Autodesk Inventor part; units mm, degrees
ref_plane "YZ Plane" through (0, 0, 0) normal (1, 0, 0) x (0, 1, 0)
ref_plane "XZ Plane" through (0, 0, 0) normal (0, 1, 0) x (-1, 0, 0)
ref_plane "XY Plane" through (0, 0, 0) normal (0, 0, 1) x (1, 0, 0)
sketch "Sketch1" plane through (0, 0, 0) normal (0, 1, 0) x (-1, 0, 0)
  line L0 (15.875, 38.1) -> (-15.875, 38.1)
  line L1 (-25.4, 28.575) -> (-25.4, -28.575)
  line L2 (-15.875, -38.1) -> (15.875, -38.1)
  line L3 (25.4, -28.575) -> (25.4, 28.575)
  line L4 (25.4, 38.1) -> (-25.4, -38.1) construction
  line L5 (-25.4, 38.1) -> (25.4, -38.1) construction
  arc A0 (15.875, -38.1) -> (25.4, -28.575) centre (15.875, -28.575) ccw
  arc A1 (25.4, 28.575) -> (15.875, 38.1) centre (15.875, 28.575) ccw
  arc A2 (-15.875, 38.1) -> (-25.4, 28.575) centre (-15.875, 28.575) ccw
  arc A3 (-25.4, -28.575) -> (-15.875, -38.1) centre (-15.875, -28.575) ccw
  line L6 (15.875, -34.925) -> (-15.875, -34.925)
  arc A4 (-22.225, -28.575) -> (-15.875, -34.925) centre (-15.875, -28.575) ccw
  line L7 (-22.225, -28.575) -> (-22.225, 28.575)
  arc A5 (-15.875, 34.925) -> (-22.225, 28.575) centre (-15.875, 28.575) ccw
  line L8 (-15.875, 34.925) -> (15.875, 34.925)
  arc A6 (22.225, 28.575) -> (15.875, 34.925) centre (15.875, 28.575) ccw
  line L9 (22.225, 28.575) -> (22.225, -28.575)
  arc A7 (15.875, -34.925) -> (22.225, -28.575) centre (15.875, -28.575) ccw
  point P0 (0, 0)
  dimension "d0" = 76.2
  dimension "d1" = 50.8
  dimension "d2" = 9.525
  dimension "d3" = 3.175
extrude "Extrusion1" add sketch "Sketch1" along normal blind 955.1356
sketch "Sketch2" plane through (-25.4, 0, -28.575) normal (-1, 0, 0) x (0, 0, 1)
  line L0 (0, 955.1356) -> (-9.525, 955.1356)
  line L1 (-9.525, 955.1356) -> (66.675, 471.8415)
  line L2 (66.675, 0) -> (66.675, 955.1356)
  line L3 (66.675, 471.8415) -> (66.675, 955.1356)
  line L4 (66.675, 955.1356) -> (-9.525, 955.1356)
  line L5 (-9.525, 0) -> (-9.525, 955.1356)
  point P0 (28.575, 0)
  dimension "d6" = 8.96
extrude "Extrusion2" cut sketch "Sketch2" against normal through all
equation "\"d0\" = stockWidth"
equation "\"d1\" = stockHeight"
equation "\"d2\" = stockRad"
equation "\"d3\" = stockGuage"
equation "\"d4\" = supVertLen"
equation "\"d6\" = sup2Ang"
equation "\"height\" = 203.2"
equation "\"shaftDiam\" = 6.35"
equation "\"shaftSpace\" = 1.5875"
equation "\"stageSpace\" = 2.54"
equation "\"stageAngle\" = 15deg"
equation "\"stockHeight\" = 50.8"
equation "\"stockWidth\" = 76.2"
equation "\"stockRad\" = 9.525"
equation "\"stockGuage\" = 3.175"
equation "\"groundActu\" = 304.8"
equation "\"baseWidth\" = 1066.8"
equation "\"baseDepth\" = 254"
equation "\"capThickness\" = 3.175"
equation "\"sup1Len\" = 660.4"
equation "\"sup1Ang\" = 22.619865deg"
equation "\"sup2Len\" = 2079.37366"
equation "\"sup2Ang\" = 8.95995deg"
equation "\"supVertLen\" = 955.13561"
equation "\"supSideAng\" = 19.376933deg"
equation "\"supSideLen\" = 1531.12879"
equation "\"FlangeDiam\" = 12.7"
equation "\"bearingDiam\" = 9.5504"
equation "\"FlangeDepth\" = 1.5875"
equation "\"smallFilet\" = 0.39687"
equation "\"thickness\" = 12.7"
equation "\"ringDiam\" = 96.46608"
properties part number "vert support" material "Aluminum 6061"
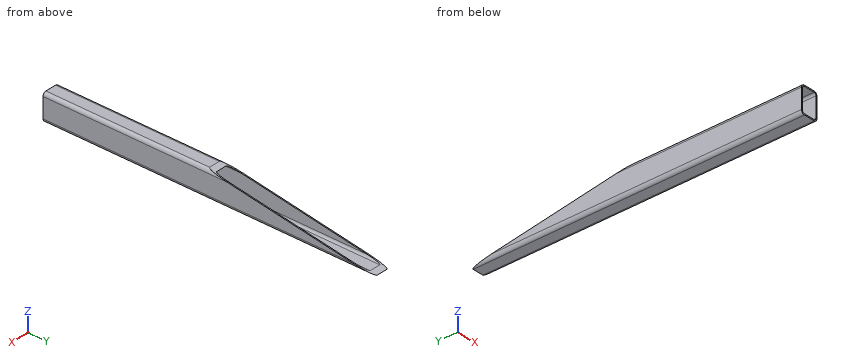
Geometry check sheet. Reference: the model listing, model coordinates, mm. Round coordinates to 2 decimals unless told otherwise and drop trailing zeros. Loops run counter-clockwise (first coordinate to the right, second up) from the corner with the lowest first, then second, coordinate; pieces in that order, holes last.
Item 1: Gauge pin test, flat end, axial feed: pin 1 (6 mm diameter, centred on x = 12.5, y = 698, fed in from +Z) (3 decimals). Record the tip position at first contact, or that the pin passes through.
Item 2: Cross-section at A-A on x = -7. Record the boundary of the cut face in (y, z) (1 decimal), then the cut area to 3 significant figures.
Item 3: Thickness scan on line 1 (X direction, y = 465, z = 24.5) (3 decimals); line 2 (Z direction, x = 10.5, y = 295.5) (3 decimals); line 3 (Z direction, x = -19, y = 68). Record the ranges inside material, lowest first.
Item 4: Cross-section at D-D on y = 676. Record the boundary of the cut face in (x, z) (3 decimals), then the cut area to 3 significant figures.
Item 5: Cross-section at C-C on z = -15.5. Record the boundary of the cut face in (x, y) (3 decimals), then the cut area to 3 significant figures.
Item 6: Cross-section at B-B on y = 194. Record the boundary of the cut face in (x, z) (3 decimals), then the cut area to 3 significant figures.
Answer sheet:
1. pin 1: stops at z = -34.925
2. outline: (0, -38.1) - (955.1, -38.1) - (935, -34.9) - (0, -34.9) - close; (0, 34.9) - (492, 34.9) - (471.8, 38.1) - (0, 38.1) - close
2. area: 4,530 mm2
3. line 1: x = -25.4 to -22.225, 22.225 to 25.4
3. line 2: z = -38.1 to -34.925, 34.925 to 38.1
3. line 3: z = -37.57 to -34.1, 34.1 to 37.57
4. outline: (-25.4, -28.575) arc R9.525 ccw to (-15.875, -38.1) - (15.875, -38.1) arc R9.525 ccw to (25.4, -28.575) - (25.4, 5.911) - (22.225, 5.911) - (22.225, -28.575) arc R6.35 cw to (15.875, -34.925) - (-15.875, -34.925) arc R6.35 cw to (-22.225, -28.575) - (-22.225, 5.911) - (-25.4, 5.911) - close
4. area: 399 mm2
5. outline: (-25.4, 0) - (-22.225, 0) - (-22.225, 811.796) - (-25.4, 811.796) - close; (22.225, 0) - (25.4, 0) - (25.4, 811.796) - (22.225, 811.796) - close
5. area: 5,150 mm2
6. outline: (-25.4, -28.575) arc R9.525 ccw to (-15.875, -38.1) - (15.875, -38.1) arc R9.525 ccw to (25.4, -28.575) - (25.4, 28.575) arc R9.525 ccw to (15.875, 38.1) - (-15.875, 38.1) arc R9.525 ccw to (-25.4, 28.575) - close; hole (-22.225, -28.575) arc R6.35 ccw to (-15.875, -34.925) - (15.875, -34.925) arc R6.35 ccw to (22.225, -28.575) - (22.225, 28.575) arc R6.35 ccw to (15.875, 34.925) - (-15.875, 34.925) arc R6.35 ccw to (-22.225, 28.575) - close
6. area: 723 mm2
